Can you work these out from the drawing? Everything is in mm from the part's minimum corner. A direction names the side the tool comes from. Coordinates: 2 decimals unless noted, no trailing zeros. Order: outer loops, then holes, each group sorted by start corner. A loop starts at its lowest first (then second) coordinate and runs counter-clockwise, first axis right, second up. Notation, with made-up numbers: (-26.75, 55) - (26.25, 55) arc R16 ccw to (26.25, 84) - close; hole circle Ø11 at (12.25, 20). An arc over 180 degrees is marked (long way). Use one line per item in the form item = value. Start each with the question number.
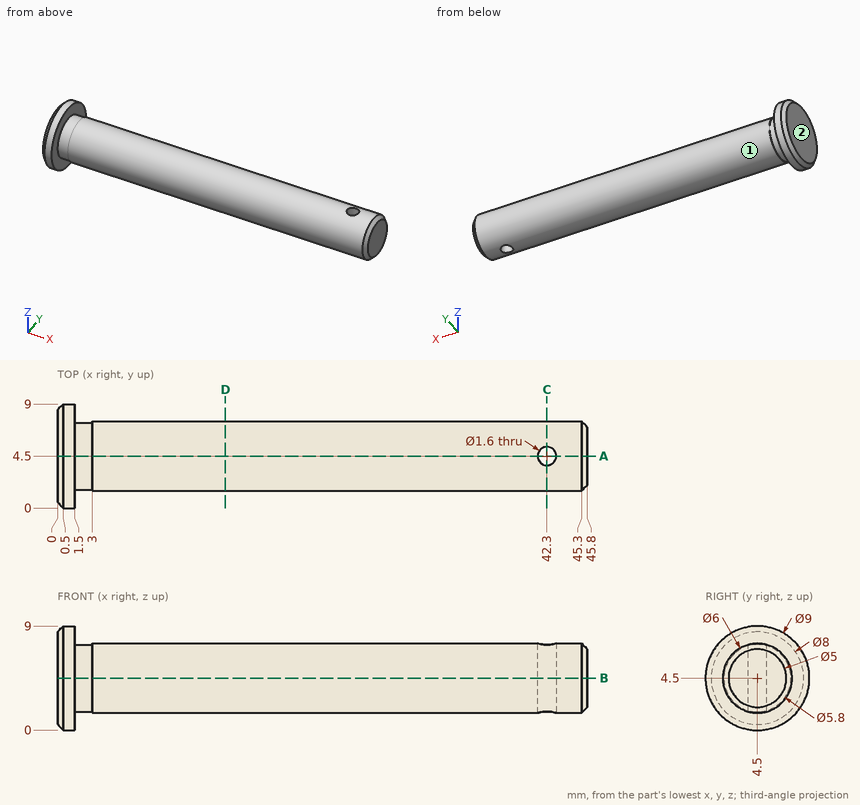
1) Suppose I cut it at B-B, the plane z = 4.5. List the corners of the cut face in (x, y) for me.
2) For pin 1 (3 mm diameter, centred on x = 15.5, z = 4.5, fed in from -Y); pin 2 (3 mm diameter, centred on x = 34.5, y = 7.5, fed in from -Z); pin 3 (2 mm diameter, centred on x = 42.3, y = 4.5, fed in from -Z); pin 4 (5 mm diameter, centred on y = 3.5, z = 5.5, fed in from -X), each with a flat end and sliding along its axis, tell me the tip position at first contact or that it passes through.
3) Suppose I cut it at C-C, the plane x = 42.3. List the corners of the cut face in (y, z) for me, then the cut area to 3 significant figures.
4) Which directions (+Z, -Z, +X, -X, +Y, -Y) give clear straight access to the entire face, cutting with the end or side of a thin tool? Please do the marked faces 1 and 2.
5) Suppose I cut it at A-A, the plane y = 4.5. List the corners of the cut face in (x, z) for me, then the cut area to 3 significant figures.
6) I need wall thicknesses on probe 1 along X at (y, z) = (4.5, 4); probe 2 along X at (y, z) = (7.25, 7.25); probe 3 along Z at (x, y) = (14, 5.25). Which ranges of each line are inside material? Lowest first, please. Write a range as [from, to].
7) Suppose I cut it at D-D, the plane x = 14.5. List the corners of the cut face in (y, z) for me.
From the geometry:
q1.outline = (0, 0.5) - (0.5, 0) - (1.5, 0) - (1.5, 1.6) - (3, 1.6) - (3, 1.5) - (45.3, 1.5) - (45.8, 2) - (45.8, 7) - (45.3, 7.5) - (3, 7.5) - (3, 7.4) - (1.5, 7.4) - (1.5, 9) - (0.5, 9) - (0, 8.5) - close; hole circle Ø1.6 at (42.3, 4.5)
q2.pin_1 = 1.5
q2.pin_2 = 1.9
q2.pin_3 = 1.5
q2.pin_4 = 0
q3.outline = (3.7, 1.61) - (3.7, 7.39) arc R3 ccw to start; (5.3, 1.61) arc R3 ccw to (5.3, 7.39) - close
q3.area = 18.8 mm2
q4.face_1 = +X
q4.face_2 = +Z, -Z, -X, +Y, -Y
q5.outline = (0, 0.5) - (0.5, 0) - (1.5, 0) - (1.5, 1.6) - (3, 1.6) - (3, 1.5) - (41.5, 1.5) - (41.5, 7.5) - (3, 7.5) - (3, 7.4) - (1.5, 7.4) - (1.5, 9) - (0.5, 9) - (0, 8.5) - close; (43.1, 1.5) - (45.3, 1.5) - (45.8, 2) - (45.8, 7) - (45.3, 7.5) - (43.1, 7.5) - close
q5.area = 269 mm2
q6.probe_1 = [0, 41.5], [43.1, 45.8]
q6.probe_2 = [0, 1.5]
q6.probe_3 = [1.6, 7.4]
q7.outline = circle Ø6 at (4.5, 4.5)
